Geometry: final body of the model. Coordinates: model frame, mm. Face numbers are marked on the shaded views. A direction names the side the tool comes from. Round coordinates to 2 decimals unless told otherwise and drop trailing zeros. Loops run counter-clockwise (first coordinate to the right, second up) from the corner with the lowest first, then second, coordinate; pieces in that order, holes last. Notation, with made-up numbers: M 8,70.25 L 34,70.25 A35 ccw 34,106.25 Z; hole C 9.25,46 d5. An arc over 180 degrees is marked long. Return JSON: item names as keys, results as strings.
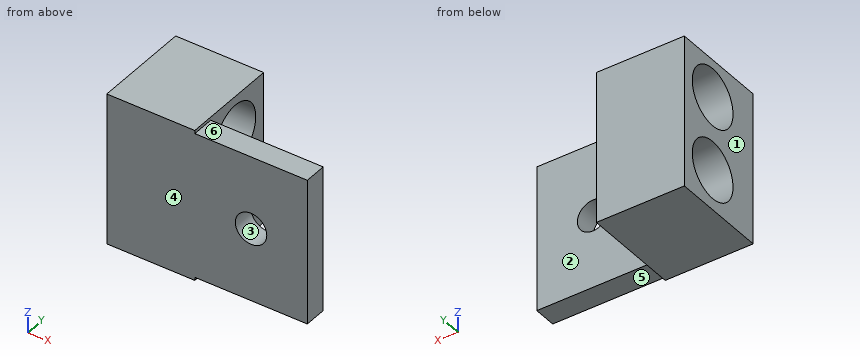
from build123d import *

# Parameters (mm, degrees)
SKETCH1_W           = 81.026
SKETCH1_H           = 39.624
BOSS_EXTRUDE1_DEPTH = 61.468
SKETCH5_W           = 45.466
SKETCH5_H           = 30.48
CUT_EXTRUDE1_DEPTH  = 62.468
SKETCH6_W           = 45.466
SKETCH6_H           = 1.27
CUT_EXTRUDE2_DEPTH  = 10.144
SKETCH7_R           = 6.35
CUT_EXTRUDE3_DEPTH  = 10.144
SKETCH8_R           = 11.7221
CUT_EXTRUDE4_DEPTH  = 36.56


with BuildPart() as part:
    # Sketch1 → Boss-Extrude1 (new body)
    with BuildSketch(Plane.XY):
        with Locations((40.513, 19.812)):
            Rectangle(SKETCH1_W, SKETCH1_H)
    extrude(amount=-BOSS_EXTRUDE1_DEPTH)

    # Sketch5 → Cut-Extrude1 (cut, through all)
    with BuildSketch(Plane.XY):
        with Locations((58.293, 24.384)):
            Rectangle(SKETCH5_W, SKETCH5_H)
    extrude(amount=-CUT_EXTRUDE1_DEPTH, mode=Mode.SUBTRACT)

    # Sketch6 → Cut-Extrude2 (cut, through all)
    with BuildSketch(Plane(origin=(0, 9.144, 0), x_dir=(1, 0, 0), z_dir=(0, 1, 0))):
        with Locations((58.293, 0.635)):
            Rectangle(SKETCH6_W, SKETCH6_H)
        with Locations((58.293, 60.833)):
            Rectangle(SKETCH6_W, SKETCH6_H)
    extrude(amount=-CUT_EXTRUDE2_DEPTH, mode=Mode.SUBTRACT)

    # Sketch7 → Cut-Extrude3 (cut, through all)
    with BuildSketch(Plane(origin=(0, 9.144, 0), x_dir=(1, 0, 0), z_dir=(0, 1, 0))):
        with Locations((58.293, 30.734)):
            Circle(SKETCH7_R)
    extrude(amount=-CUT_EXTRUDE3_DEPTH, mode=Mode.SUBTRACT)

    # Sketch8 → Cut-Extrude4 (cut, through all)
    with BuildSketch(Plane(origin=(35.56, 0, 0), x_dir=(0, 0, -1), z_dir=(1, 0, 0))):
        with Locations((15.307348572, 23.33723476)):
            Circle(SKETCH8_R)
        with Locations((45.18450858, 23.33723476)):
            Circle(SKETCH8_R)
    extrude(amount=-CUT_EXTRUDE4_DEPTH, mode=Mode.SUBTRACT)


solid = part.part
Q1. Section query D-D (z = -26). Output: boundary loops of the cut face in (x, y), plus the area to 3 significant figures.
Determined:
{"outline": "M 0,0 L 54.06,0 L 54.06,9.14 L 35.56,9.14 L 35.56,18.53 L 0,18.53 Z; M 0,28.14 L 35.56,28.14 L 35.56,39.62 L 0,39.62 Z; M 62.53,0 L 81.03,0 L 81.03,9.14 L 62.53,9.14 Z", "area": "1,410 mm^2"}
Q2. Section query B-B (y = 20.5). Output: boundary loops of the cut face in (x, z).
Determined:
{"outline": "M 0,-61.47 L 35.56,-61.47 L 35.56,-56.56 L 0,-56.56 Z; M 0,-33.81 L 35.56,-33.81 L 35.56,-26.68 L 0,-26.68 Z; M 0,-3.93 L 35.56,-3.93 L 35.56,0 L 0,0 Z"}
Q3. Section query C-C (x = 55). Output: boundary loops of the cut face in (y, z).
Determined:
{"outline": "M 0,-60.2 L 9.14,-60.2 L 9.14,-36.16 L 0,-36.16 Z; M 0,-25.3 L 9.14,-25.3 L 9.14,-1.27 L 0,-1.27 Z"}
Q4. Section query A-A (z = -42.5). Output: boundary loops of the cut face in (x, y), plus the area to 3 significant figures.
Determined:
{"outline": "M 0,0 L 81.03,0 L 81.03,9.14 L 35.56,9.14 L 35.56,11.93 L 0,11.93 Z; M 0,34.75 L 35.56,34.75 L 35.56,39.62 L 0,39.62 Z", "area": "1,010 mm^2"}
Q5. Pull-direction query (X, two-part tool) for the marked faces 1, 2 and 3; classes: pulls with the +X half, pulls with the -X half, needs draft (parallel to the pull), parting line crosses it, or undercut.
Determined:
{"face 1": "pulls with the -X half", "face 2": "needs draft", "face 3": "undercut"}
Q6. Reachability of the marked faces 4, 5 and 6 from +Z, -Z, +X, -X, +Y, -Y: full face, straight path, thin tool, end or side. Return the list, or none.
Determined:
{"face 4": "+Z, -Z, +X, -X, -Y", "face 5": "-Z, +X, +Y, -Y", "face 6": "+Z, +X, +Y, -Y"}
Q7. Material intervals for L1, parallel to Z at x = 19.5, y = 25; L2, parallel to Z at x = 8, y = 13.5; L3, parallel to X at y = 35, z = -42.5, sorted ascending.
Determined:
{"L1": "z = -61.47 to -56.79, -33.58 to -26.91, -3.7 to 0", "L2": "z = -61.47 to -51.56, -38.81 to -21.68, -8.93 to 0", "L3": "x = 0 to 35.56"}
Q8. Pin query (flat end, axial travel): pin 1 (10 mm diameter, centred on x = 61.5, y = 6.5, fed in from -Z); pin 2 (2.5 mm diameter, centred on x = 62.5, y = 5.5, fed in from +Z); pin 3 (5 mm diameter, centred on y = 25.5, z = -33, fed in from -X); pin 4 (11.5 mm diameter, centred on x = 58.293, z = -30.734, fed in from -Y). Return the tip coordinate at first contact, or that it passes through.
Determined:
{"pin 1": "stops at z = -60.2", "pin 2": "stops at z = -1.27", "pin 3": "stops at x = 0", "pin 4": "passes through"}
